Design review of the part shown in the three views and the two pictorial views. Dimensions are in mm from the part's minimum x, y and z. A direction names the side the tool comes from. Round coordinates to 2 decimals unless told otherwise and drop trailing zeros. Order: outer loops, then holes, each group sorted by start corner. A loop starts at its lowest first (then second) coordinate and runs counter-clockwise, first axis right, second up. Notation, with made-up numbers: (-20, 60) - (2, 60) arc R28 cw to (2, 80) - close; hole circle Ø2 at (43, 71.25). An arc over 180 degrees is marked (long way). One line per question, with ' | ' between items. Start each with the question number.
Item 1: Insertion check: pin 1 Ø1.5 at (y, z) = (26, 33) entering from -X; pin 2 Ø9.5 at (x, y) = (107, 26.5) entering from +Z; pin 3 Ø1 at (x, z) = (51, 17) entering from +Y. Each pin has a flat end and moves straight along its axis. Give the tip position at first contact, or say it passes through.
Item 2: Add section C-C on y = 32. State the section outline as (x, z) points, and give its area (3 significant figures).
Item 3: Add section D-D on z = 6.5. State the section outline as (x, y) points (1 decimal), and give its area (3 significant figures).
Item 4: For L1, parallel to Z at x = 63, y = 31; L2, parallel to X at y = 58, z = 33; L3, parallel to X at y = 37.5, z = 29.5, list the stretches that pass through material, from the lowest coordinate up. Write a range as [from, to].
Item 5: Tool access review of the marked faces 4, 5, 6, 7 and 8: name each direction out of +Z, -Z, +X, -X, +Y, -Y from which nothing blocks a thin tool from reaching the whole face with its end or side.
Item 6: Add section B-B on x = 63.5. State the section outline as (y, z) points.
Item 7: Add section A-A on z = 44. State the section outline as (x, y) points, and give its area (3 significant figures).
Item 8: Draft analysis for pull direction Y (two halves, no side actions). For the marked faces 1, 2 and 3, state which applies: +Y half, -Y half, draft (parallel to the pull), parting line (faces both ways), or undercut.
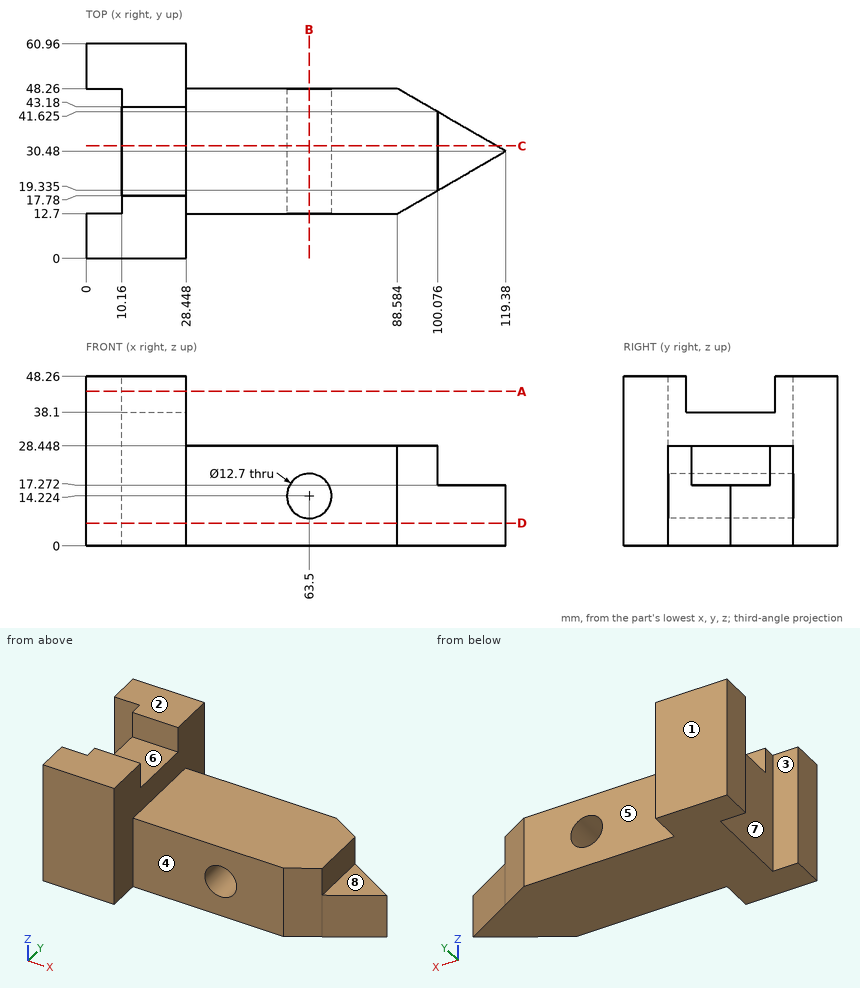
Determined:
1) pin 1: x = 10.16 | pin 2: z = 17.27 | pin 3: y = 48.26
2) outline: (10.16, 0) - (116.75, 0) - (116.75, 17.27) - (100.08, 17.27) - (100.08, 28.45) - (28.45, 28.45) - (28.45, 38.1) - (10.16, 38.1) - close; hole circle Ø12.7 at (63.5, 14.22) | area: 2,900 mm2
3) outline: (0, 0) - (28.4, 0) - (28.4, 12.7) - (88.6, 12.7) - (119.4, 30.5) - (88.6, 48.3) - (28.4, 48.3) - (28.4, 61) - (0, 61) - (0, 48.3) - (10.2, 48.3) - (10.2, 12.7) - (0, 12.7) - close | area: 4,060 mm2
4) L1: [0, 7.89], [20.55, 28.45] | L2: [0, 28.45] | L3: [10.16, 28.45]
5) face 4: +Z, -Z, +X, -Y | face 5: +Z, -Z, +X, +Y | face 6: +Z, +X, -X | face 7: +Z, -Z, -X | face 8: +Z, +X, +Y, -Y
6) outline: (12.7, 0) - (48.26, 0) - (48.26, 7.87) - (12.7, 7.87) - close; (12.7, 20.57) - (48.26, 20.57) - (48.26, 28.45) - (12.7, 28.45) - close
7) outline: (0, 0) - (28.45, 0) - (28.45, 17.78) - (10.16, 17.78) - (10.16, 12.7) - (0, 12.7) - close; (0, 48.26) - (10.16, 48.26) - (10.16, 43.18) - (28.45, 43.18) - (28.45, 60.96) - (0, 60.96) - close | area: 908 mm2
8) face 1: +Y half | face 2: draft | face 3: undercut
